Geometry check sheet. Reference: the model listing, model coordinates, mm. A direction names the side the tool comes from. Round coordinates to 2 decimals unless told otherwise and drop trailing zeros. Write each loop counter-clockwise with the first axis right and the second up, starting at its lowest first coordinate (ties: lowest second). Pieces come first, ordered by that corner, then holes. Notation, with made-up numbers: (-29.75, 52) - (27.25, 52) arc R5 ccw to (27.25, 57) - close; hole circle Ø4 at (6, 28.25). An arc over 180 degrees is marked (long way). One line per question, with ' | ' between items. Start each with the question number.
from build123d import *

# Parameters (mm, degrees)
SKETCH1_R            = 5.3975
BOSS_EXTRUDE1_DEPTH  = 1.651
SKETCH2_R            = 8.509
BOSS_EXTRUDE2_DEPTH  = 5.842
SKETCH3_R            = 3.429
BOSS_EXTRUDE3_DEPTH  = 6.35
SKETCH6_R            = 2.9845
BOSS_EXTRUDE5_DEPTH  = 13.462
SKETCH12_W           = 6.35
SKETCH12_H           = 1.016
CUT_EXTRUDE1_DEPTH   = 11.176
BOSS_EXTRUDE7_DEPTH  = 1.27
SKETCH14_R           = 1.524
BOSS_EXTRUDE11_DEPTH = 1.016
LPATTERN2_START      = -3.302
LPATTERN2_OUTLINE_R  = 1.524
LPATTERN2_DEPTH      = 2.032
LPATTERN2_START_2    = -1.651
LPATTERN2_2_DEPTH    = 0.381
SKETCH4_R            = 1.397
BOSS_EXTRUDE8_DEPTH  = 3.81


# Read off the part's stored shape, not the designer's step: LPattern2
with BuildPart() as part:
    # Sketch1 → Boss-Extrude1 (new body)
    with BuildSketch(Plane(origin=(0, 0, 0), x_dir=(1, 0, 0), z_dir=(0, 1, 0))):
        with Locations(Location((0, 0, 0), (0, 0, 270))):
            Circle(SKETCH1_R)
    extrude(amount=-BOSS_EXTRUDE1_DEPTH)

    # Sketch2 → Boss-Extrude2 (add)
    with BuildSketch(Plane.XZ.offset(1.651)):
        with Locations(Location((0, 0, 0), (0, 0, 270))):
            Circle(SKETCH2_R)
    extrude(amount=BOSS_EXTRUDE2_DEPTH)

    # Sketch3 → Boss-Extrude3 (add)
    with BuildSketch(Plane(origin=(0, 0, 0), x_dir=(1, 0, 0), z_dir=(0, 1, 0))):
        with Locations(Location((0, 0, 0), (0, 0, 270))):
            Circle(SKETCH3_R)
    extrude(amount=BOSS_EXTRUDE3_DEPTH)

    # Sketch6 → Boss-Extrude5 (add)
    with BuildSketch(Plane(origin=(0, 6.35, 0), x_dir=(1, 0, 0), z_dir=(0, 1, 0))):
        with Locations(Location((0, 0, 0), (0, 0, 270))):
            Circle(SKETCH6_R)
    extrude(amount=BOSS_EXTRUDE5_DEPTH)

    # Sketch12 → Cut-Extrude1 (cut)
    with BuildSketch(Plane(origin=(0, 19.812, 0), x_dir=(1, 0, 0), z_dir=(0, 1, 0))):
        Rectangle(SKETCH12_W, SKETCH12_H)
    extrude(amount=-CUT_EXTRUDE1_DEPTH, mode=Mode.SUBTRACT)

    # Sketch11 → Boss-Extrude7 (add)
    with BuildSketch(Plane.XZ.offset(1.651)):
        with BuildLine():
            Line((-7.62, 3.175), (-7.62, 11.557))
            Line((-7.62, 11.557), (7.62, 11.557))
            Line((7.62, 11.557), (7.62, 3.175))
            ThreePointArc((7.62, 3.175), (0, -8.255), (-7.62, 3.175))
        make_face()
    extrude(amount=BOSS_EXTRUDE7_DEPTH)

    # Sketch14 → Boss-Extrude11 (add, symmetric)
    with BuildSketch(Plane(origin=(0, -2.286, 0), x_dir=(1, 0, 0), z_dir=(0, 1, 0))):
        with Locations(Location((-5.08, -8.509, 0), (0, 0, 90))):
            Circle(SKETCH14_R)
    extrude(amount=BOSS_EXTRUDE11_DEPTH, both=True)

    # LPattern2 outline → LPattern2 (add)
    with BuildSketch(Plane(origin=(0, 0, 0), x_dir=(1, 0, 0), z_dir=(0, 1, 0)).offset(LPATTERN2_START)):
        with Locations((0, -8.509)):
            Circle(LPATTERN2_OUTLINE_R)
        with BuildLine():
            ThreePointArc((5.330666391, -7.005756054), (4.298782485, -9.817539336), (6.284337715, -7.575112069))
            ThreePointArc((6.284337715, -7.575112069), (5.798202212, -7.306011296), (5.330666391, -7.005756054))
        make_face()
    extrude(amount=LPATTERN2_DEPTH)

    # LPattern2 2 outline → LPattern2 2 (add)
    with BuildSketch(Plane(origin=(0, 0, 0), x_dir=(1, 0, 0), z_dir=(0, 1, 0)).offset(LPATTERN2_START_2)):
        with BuildLine():
            ThreePointArc((5.330666391, -7.005756054), (5.798202212, -7.306011296), (6.284337715, -7.575112069))
            ThreePointArc((6.284337715, -7.575112069), (5.861217515, -7.200460664), (5.330666391, -7.005756054))
        make_face()
    extrude(amount=LPATTERN2_2_DEPTH)

    # Sketch4 → Boss-Extrude8 (add)
    with BuildSketch(Plane(origin=(0, -1.651, 0), x_dir=(1, 0, 0), z_dir=(0, 1, 0))):
        with Locations(Location((-7.874, 0, 0), (0, 0, 112.591863996))):
            Circle(SKETCH4_R)
    extrude(amount=BOSS_EXTRUDE8_DEPTH)


solid = part.part
Q1. Set-up check for faces 4 (the flat face through (5, -1.27, 8)), 5 (the cylindrical face through (3.648, -0.814, -3.978)), 6 (the flat face through (-8, 2.159, 0)): record each of +Z, -Z, +X, -X, +Y, -Y from which the full face is reachable in a straight line by a thin tool's end or side.
Q2. Section check A-A, the plane z = 0. Record the cut outline in (x, y), then the cut area to 3 significant figures.
Q3. Section check C-C, the plane y = 14.5. Record the cut outline in (x, z), then the cut area to 3 significant figures.
Q4. Thickness scan on line 1 (Y direction, x = 0, z = 9.25); line 2 (Y direction, x = -3.25, z = -4.5); line 3 (Z direction, x = 1.5, y = -6). Record the ranges inside material, lowest first.
Q5. Go/stop test with flat-tipped pins: P1, Ø0.9, axis at x = 0.5, z = 8.5, coming from the +Y side; P2, Ø8, axis at x = 5.5, y = 8.5, coming from the -Z side; P3, Ø0.6, axis at y = -2, z = 6, coming from the -X side. Record where each tip stops, or that it passes through.
Q6. Section check D-D, the plane y = 3.5. Record the cut outline in (x, z).
Q7. Draft check along X on faces 1 (the flat face through (-5, -1.27, 9)), 2 (the cylindrical face through (-2.648, 12.987, 1.377)), 3 (the cylindrical face through (-0.035, -3.114, 10.033)). Enter one of: pulls with the +X half, pulls with the -X half, needs draft (parallel to the pull), parting line crosses it, or undercut.
Result sheet:
1) face 4: +Z, +X, -X, +Y | face 5: +Y | face 6: +Z, -Z, -X, +Y
2) outline: (-9.27, -1.65) - (-8.51, -1.65) - (-8.51, -7.49) - (8.51, -7.49) - (8.51, -1.65) - (5.4, -1.65) - (5.4, 0) - (3.43, 0) - (3.43, 6.35) - (2.98, 6.35) - (2.98, 8.64) - (-2.98, 8.64) - (-2.98, 6.35) - (-3.43, 6.35) - (-3.43, 0) - (-5.4, 0) - (-5.4, -1.65) - (-6.48, -1.65) - (-6.48, 2.16) - (-9.27, 2.16) - close | area: 185 mm²
3) outline: (-2.94, -0.51) arc R2.98 ccw to (2.94, -0.51) - close; (-2.94, 0.51) - (2.94, 0.51) arc R2.98 ccw to start | area: 21.9 mm²
4) line 1: -3.3 to -1.27 | line 2: -7.49 to -1.65 | line 3: -8.38 to 8.38
5) P1: y = -1.27 | P2: z = -2.69 | P3: x = -7.62
6) outline: circle Ø6.86 at (0, 0)
7) face 1: needs draft | face 2: parting line crosses it | face 3: undercut
